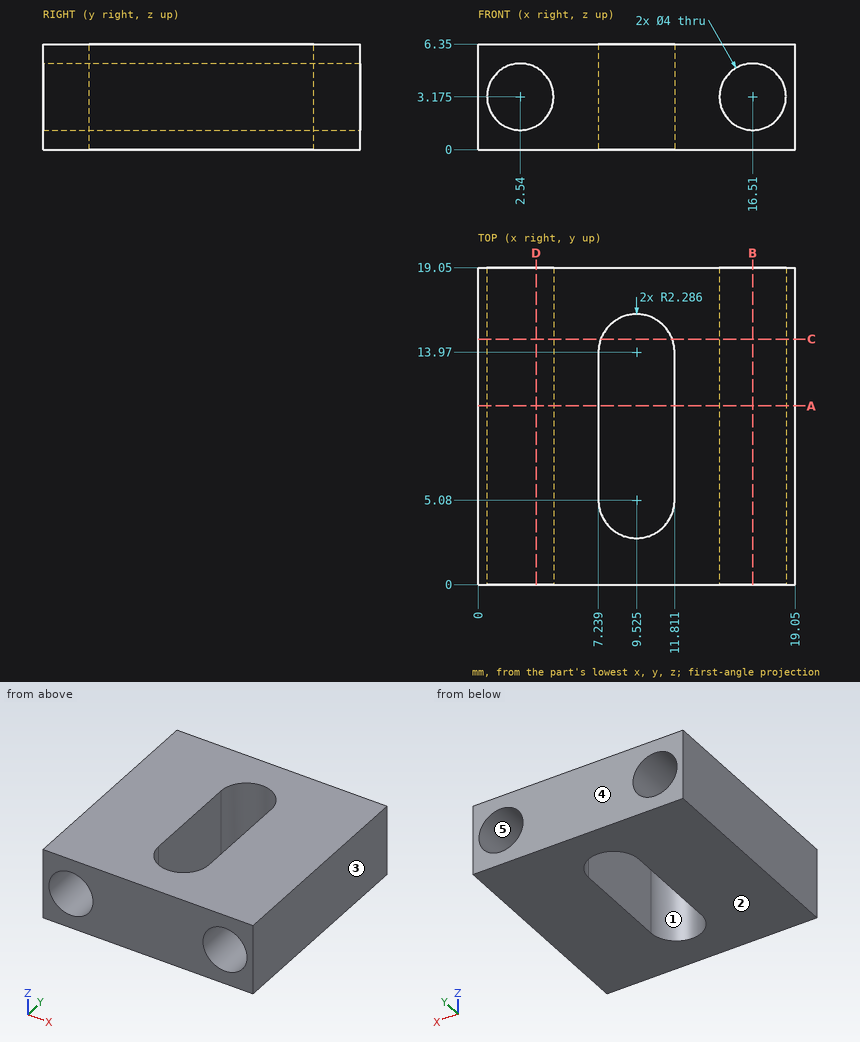
For this review, use the dimensioned drawing (mm, ordinates from the lowest corner) and the shaded views. A direction names the side the tool comes from. Coordinates: 2 decimals unless noted, no trailing zeros. Order: outer loops, then holes, each group sorted by start corner. A loop starts at its lowest first (then second) coordinate and runs counter-clockwise, first axis right, second up. Notation, with made-up numbers: (-23, -22.5) -> (2, -22.5) arc R19 cw to (2, 7.5) -> close; hole circle Ø11 at (67.25, 40.25). An arc over 180 degrees is marked (long way). One line per item, written item: value. Start each with the question number.
Q1. For probe 1 along X at (y, z) = (10.25, 3); probe 2 along Z at (x, y) = (16.5, 17.75); probe 3 along X at (y, z) = (16.5, 2), list the stretches that pass through material, from the lowest coordinate up.
Q2. Mouldability with a two-part tool opening along X and no side actions: class the marked faces 3, 4 and 5 as pulls with the +X half, pulls with the -X half, needs draft (parallel to the pull), parting line crosses it, or undercut.
Q3. Take a section at A-A, the plane y = 10.75. State the section outline as (x, z) points (3 decimals).
Q4. Take a section at C-C, the plane y = 14.75. State the section outline as (x, z) points (3 decimals).
Q5. Take a section at B-B, the plane x = 16.51. State the section outline as (y, z) points (3 decimals).
Q6. Tool access review of the marked faces 1 and 2: name each direction out of +Z, -Z, +X, -X, +Y, -Y from which nothing blocks a thin tool from reaching the whole face with its end or side.
Q7. Insertion check: pin 1 Ø3 at (x, z) = (16.51, 3.175) entering from +Y (3 decimals). The pin has a flat end and moves straight along its axis. Give the tip position at first contact, or say it passes through.
Q8. Take a section at D-D, the plane x = 3.5. State the section outline as (y, z) points, then the cut area to 3 significant figures.
Values follow:
1. probe 1: x = 0 to 0.55, 4.53 to 7.24, 11.81 to 14.52, 18.5 to 19.05
1. probe 2: z = 0 to 1.18, 5.17 to 6.35
1. probe 3: x = 0 to 0.92, 4.16 to 14.89, 18.13 to 19.05
2. face 3: pulls with the +X half
2. face 4: needs draft
2. face 5: undercut
3. outline: (0, 0) -> (7.239, 0) -> (7.239, 6.35) -> (0, 6.35) -> close; (11.811, 0) -> (19.05, 0) -> (19.05, 6.35) -> (11.811, 6.35) -> close; hole circle Ø4 at (2.54, 3.175); hole circle Ø4 at (16.51, 3.175)
4. outline: (0, 0) -> (7.376, 0) -> (7.376, 6.35) -> (0, 6.35) -> close; (11.674, 0) -> (19.05, 0) -> (19.05, 6.35) -> (11.674, 6.35) -> close; hole circle Ø4 at (2.54, 3.175); hole circle Ø4 at (16.51, 3.175)
5. outline: (0, 0) -> (19.05, 0) -> (19.05, 1.175) -> (0, 1.175) -> close; (0, 5.175) -> (19.05, 5.175) -> (19.05, 6.35) -> (0, 6.35) -> close
6. face 1: +Z, -Z
6. face 2: -Z, +X, -X, +Y, -Y
7. pin 1: passes through
8. outline: (0, 0) -> (19.05, 0) -> (19.05, 1.42) -> (0, 1.42) -> close; (0, 4.93) -> (19.05, 4.93) -> (19.05, 6.35) -> (0, 6.35) -> close
8. area: 54.1 mm2
